from build123d import *

# Parameters (mm, degrees)
SKETCH_1_W             = 20
SKETCH_1_H             = 28.9
EXTRUDE_1_DEPTH        = 8
SKETCH_2_W             = 9
SKETCH_2_H             = 4.5
CUT_EXTRUDE_1_DEPTH    = 29.9
HOLE_WIZARD_M3_1_D     = 2.5
HOLE_WIZARD_M3_1_DEPTH = 10.1
HOLE_WIZARD_M3_1_TIP   = 0.751075774


with BuildPart() as part:
    # 草图1 → 凸台-拉伸1 (new body)
    with BuildSketch(Plane.XY):
        with Locations((10, 14.45)):
            Rectangle(SKETCH_1_W, SKETCH_1_H)
    extrude(amount=EXTRUDE_1_DEPTH)

    # 草图2 → 切除-拉伸1 (cut, through all)
    with BuildSketch(Plane(origin=(0, 28.9, 0), x_dir=(1, 0, 0), z_dir=(0, 1, 0))):
        with Locations((10, -5.75)):
            Rectangle(SKETCH_2_W, SKETCH_2_H)
    extrude(amount=-CUT_EXTRUDE_1_DEPTH, mode=Mode.SUBTRACT)

    # M3 螺纹孔1
    with Locations(Plane(origin=(0, 0, 0), x_dir=(-1, 0, 0), z_dir=(0, 0, -1))):
        with Locations((-2.5, 9.45), (-17.5, 9.45), (-2.5, 19.45), (-17.5, 19.45)):
            Hole(HOLE_WIZARD_M3_1_D / 2, depth=HOLE_WIZARD_M3_1_DEPTH)
            with Locations((0, 0, -(HOLE_WIZARD_M3_1_DEPTH + HOLE_WIZARD_M3_1_TIP / 2))):  # 118° drill point
                Cone(0, HOLE_WIZARD_M3_1_D / 2, HOLE_WIZARD_M3_1_TIP, mode=Mode.SUBTRACT)


solid = part.part
CAD build for the part. Positions are in the model's coordinates, mm. A direction names the side the tool comes from. Round coordinates to 2 decimals unless told otherwise and drop trailing zeros. Loops run counter-clockwise (first coordinate to the right, second up) from the corner with the lowest first, then second, coordinate; pieces in that order, holes last. Notation, with made-up numbers: (74, 37.5) - (100, 37.5) arc R25 ccw to (100, 75.5) - close; hole circle Ø1 at (78, -22). An arc over 180 degrees is marked (long way). Put each result on its own line as item: value.
1. Two-plate mould, pull along X, no slides. Class faces 3 (the flat face through (10, 15, 3.5)), 4 (the flat face through (0, 14, 4)), 5 (the flat face through (10, 15, 0)), 6 (the flat face through (14.5, 15, 6)): released by +X, released by -X, zero draft, split by the parting line, or undercut.
Geometry check:
face 3: undercut
face 4: released by -X
face 5: zero draft
face 6: undercut
2. Slice it at A-A on z = 4.25. List the corners of the cut face in (x, y).
Geometry check:
outline: (0, 0) - (5.5, 0) - (5.5, 28.9) - (0, 28.9) - close; (14.5, 0) - (20, 0) - (20, 28.9) - (14.5, 28.9) - close; hole circle Ø2.5 at (2.5, 9.45); hole circle Ø2.5 at (2.5, 19.45); hole circle Ø2.5 at (17.5, 9.45); hole circle Ø2.5 at (17.5, 19.45)
3. Wall check: line 1 (Y direction, x = 17.5, z = 3.5); line 2 (X direction, y = 9.5, z = 2.5); line 3 (X direction, y = 27, z = 6). Give the ranges that are in metal, low to high.
Geometry check:
line 1: 0 to 8.2, 10.7 to 18.2, 20.7 to 28.9
line 2: 0 to 1.25, 3.75 to 16.25, 18.75 to 20
line 3: 0 to 5.5, 14.5 to 20
4. Slice it at D-D on z = 2. List the corners of the cut face in (x, y).
Geometry check:
outline: (0, 0) - (20, 0) - (20, 28.9) - (0, 28.9) - close; hole circle Ø2.5 at (2.5, 9.45); hole circle Ø2.5 at (2.5, 19.45); hole circle Ø2.5 at (17.5, 9.45); hole circle Ø2.5 at (17.5, 19.45)
5. Slice it at C-C on x = 2.5. List the corners of the cut face in (y, z), and give its area (3 significant figures).
Geometry check:
outline: (0, 0) - (8.2, 0) - (8.2, 8) - (0, 8) - close; (10.7, 0) - (18.2, 0) - (18.2, 8) - (10.7, 8) - close; (20.7, 0) - (28.9, 0) - (28.9, 8) - (20.7, 8) - close
area: 191 mm²
6. Slice it at B-B on y = 9.45. List the corners of the cut face in (x, z).
Geometry check:
outline: (0, 0) - (1.25, 0) - (1.25, 8) - (0, 8) - close; (3.75, 0) - (16.25, 0) - (16.25, 8) - (14.5, 8) - (14.5, 3.5) - (5.5, 3.5) - (5.5, 8) - (3.75, 8) - close; (18.75, 0) - (20, 0) - (20, 8) - (18.75, 8) - close
7. 3-axis set-ups, long thin cutter, end or side, ignore diameter. For faces 1 (the flat face through (10, 0, 3)), 2 (the flat face through (5.5, 15, 6)): which of +Z, -Z, +X, -X, +Y, -Y reach the whole face in a straight line?
Geometry check:
face 1: +Z, -Z, +X, -X, -Y
face 2: +Z, +Y, -Y
8. Pin check, flat tips, straight feed: P1, Ø2.5, axis at x = 8, y = 15, coming from the +Z side; P2, Ø1.5, axis at x = 2.5, y = 19.45, coming from the +Z side. Stop position of each tip, or through.
Geometry check:
P1: z = 3.5
P2: through
